from build123d import *

# Parameters (mm, degrees)
F0_W      = 177
F0_H      = 46
F0_W_2    = 173
F0_H_2    = 38
F1_DEPTH  = 33
F2_W      = 153
F2_H      = 27
F3_DEPTH  = 6
F4_W      = 5
F4_H      = 38
F5_DEPTH  = 17
F6_W      = 13
F6_H      = 11
F7_DEPTH  = 25
F9_R      = 1.4
F10_DEPTH = 5
F11_W     = 153
F11_H     = 4
F12_DEPTH = 6


with BuildPart() as f1:
    # F0 (on Top) → F1 (new body)
    with BuildSketch(Plane.XY):
        Rectangle(F0_W, F0_H)
        with Locations((0, 2)):
            Rectangle(F0_W_2, F0_H_2, mode=Mode.SUBTRACT)
    extrude(amount=F1_DEPTH)

    # F2 (on face) → F3 (cut)
    with BuildSketch(Plane.XZ.offset(23)):
        with Locations((-2, 19.5)):
            Rectangle(F2_W, F2_H)
    extrude(amount=-F3_DEPTH, mode=Mode.SUBTRACT)

    # F4 (on Top) → F5 (join)
    with BuildSketch(Plane.XY):
        with Locations((-84, 2)):
            Rectangle(F4_W, F4_H)
        with Locations((84, 2)):
            Rectangle(F4_W, F4_H)
    extrude(amount=F5_DEPTH)

    # F6 (on face) → F7 (cut)
    with BuildSketch(Plane.YZ.offset(88.5)):
        Polygon((16, 33), (-12, 33), (-12, 20), (1, 20), (16, 20), align=None)
        with Locations((-5.5, 14.5)):
            Rectangle(F6_W, F6_H)
    extrude(amount=-F7_DEPTH, mode=Mode.SUBTRACT)

    # F9 (on offset) → F10 (cut)
    with BuildSketch(Plane.XY.offset(33)):
        with Locations((-83.5, -20)):
            Circle(F9_R)
        with Locations((83.5, -20)):
            Circle(F9_R)
    extrude(amount=-F10_DEPTH, mode=Mode.SUBTRACT)

    # F11 (on face) → F12 (cut)
    with BuildSketch(Plane.XY.offset(6)):
        with Locations((-2, -19)):
            Rectangle(F11_W, F11_H)
    extrude(amount=-F12_DEPTH, mode=Mode.SUBTRACT)


solid = f1.part
Check sheet for the modelled part. Datum: model origin and axes. Units: mm. A direction names the side the tool comes from. Give positions to 0.01 mm unless a question says otherwise; leave off trailing zeros. Loops run counter-clockwise (first coordinate to the right, second up) from the corner with the lowest first, then second, coordinate; pieces in that order, holes last. Notation, with made-up numbers: M -6,-22.75 L 43,-22.75 A3 ccw 43,-17.75 Z; hole C 76.5,-6 d3. An arc over 180 degrees is marked long. Use a Markdown table: item, result. Add a question column.
Q1. Sectioned sample at B-B, the plane y = 14. Record the cut outline in (x, z), then the cut area to 3 significant figures.
Q2. Sectioned sample at A-A, the plane z = 29.5. Record the cut outline in (x, y).
Q3. Tool access check on faces 4 (the flat face through (85, 1, 13)), 5 (the flat face through (-3, -21, 3)), 6 (the flat face through (-84, -20, 28)). Record the directions out of +Z, -Z, +X, -X, +Y, -Y that give a thin tool (end or side, any length) a straight path to the whole face; none if there is none.
Q4. Go/stop test with flat-tipped pins: pin 1 (7.5 mm diameter, centred on x = 84.5, y = -7, fed in from +Z); pin 2 (10 mm diameter, centred on x = -51.5, z = 25, fed in from -Y); pin 3 (8.5 mm diameter, centred on y = -4.5, z = 10.5, fed in from +X); pin 4 (1 mm diameter, centred on x = 87.5, y = 9, fed in from +Z). Record where each tip stops, or that it passes through.
Q5. Scan lines: line 1 along Y through (x, z) = (-83.5, 30.95); line 2 along X through (y, z) = (-6, 3.5); line 3 along Y through (x, z) = (-14.5, 4.5). Record each from-to range of solid material in increasing order. Write a range as [from, to].
Q6. Mould release check, pull along X, two halves, no side actions. Record for faces 1 (the flat face through (85, -6, 9)), 2 (the flat face through (83, -20, 28)), 3 (the flat face through (88.5, 5, 13)): pulls with the +X half, pulls with the -X half, needs draft (parallel to the pull), parting line crosses it, or undercut.
Q7. Sectioned sample at C-C, the plane x = -31.5. Record the cut outline in (y, z).
Verdict:
| question | item | result |
|---|---|---|
| 1 | outline | M -88.5,0 L -81.5,0 L -81.5,17 L -86.5,17 L -86.5,33 L -88.5,33 Z; M 81.5,0 L 88.5,0 L 88.5,20 L 86.5,20 L 86.5,17 L 81.5,17 Z |
| 1 | area | 276 mm^2 |
| 2 | outline | M -88.5,-23 L -78.5,-23 L -78.5,-17 L -86.5,-17 L -86.5,21 L 86.5,21 L 86.5,16 L 88.5,16 L 88.5,23 L -88.5,23 Z; M 74.5,-23 L 88.5,-23 L 88.5,-12 L 86.5,-12 L 86.5,-17 L 74.5,-17 Z; hole C -83.5,-20 d2.8; hole C 83.5,-20 d2.8 |
| 3 | face 4 | +Z, +X |
| 3 | face 5 | +Z, -Z |
| 3 | face 6 | +Z |
| 4 | pin 1 | z = 9 |
| 4 | pin 2 | y = 21 |
| 4 | pin 3 | x = 88.5 |
| 4 | pin 4 | z = 20 |
| 5 | line 1 | [-23, -21.4], [-18.6, -17], [21, 23] |
| 5 | line 2 | [-88.5, -81.5], [81.5, 88.5] |
| 5 | line 3 | [-23, -21], [21, 23] |
| 6 | face 1 | needs draft |
| 6 | face 2 | undercut |
| 6 | face 3 | pulls with the +X half |
| 7 | outline | M -23,0 L -21,0 L -21,6 L -23,6 Z; M 21,0 L 23,0 L 23,33 L 21,33 Z |
